```python
from build123d import *

# Parameters (mm, degrees)
F0_R     = 10.16
F1_DEPTH = 15.7734
F2_DEPTH = 40.2336
F3_R     = 3.302


with BuildPart() as f1:
    # F0 (on Top) → F1 (new body)
    with BuildSketch(Plane.XY):
        with BuildLine():
            ThreePointArc((5.403247, 28.0595), (22.033252, 18.195231), (28.575, 0))
            ThreePointArc((28.575, 0), (22.033252, -18.195231), (5.403247, -28.0595))
            Line((5.403247, -28.0595), (53.975, -18.706333))
            ThreePointArc((53.975, -18.706333), (69.422835, 0), (53.975, 18.706333))
            Line((53.975, 18.706333), (5.403247, 28.0595))
        make_face()
        with Locations((53.975, 0)):
            Circle(F0_R, mode=Mode.SUBTRACT)
    extrude(amount=F1_DEPTH)

    # F0 (on Top) → F2 (join)
    with BuildSketch(Plane.XY):
        with BuildLine():
            ThreePointArc((5.403247, -28.0595), (22.033252, -18.195231), (28.575, 0))
            ThreePointArc((28.575, 0), (22.033252, 18.195231), (5.403247, 28.0595))
            ThreePointArc((5.403247, 28.0595), (-28.575, 0), (5.403247, -28.0595))
        make_face()
        with BuildLine():
            ThreePointArc((13.447765, -4.826), (-14.2875, 0), (13.447765, 4.826))
            Line((13.447765, 4.826), (18.5293, 4.826))
            Line((18.5293, 4.826), (18.5293, 0))
            Line((18.5293, 0), (18.5293, -4.826))
            Line((18.5293, -4.826), (13.447765, -4.826))
        make_face(mode=Mode.SUBTRACT)
    extrude(amount=F2_DEPTH)

    # F3
    f3_edges = [f1.edges().sort_by_distance(p)[0] for p in [
        (-5.403247, 28.0595, 40.2336),
    ]]
    fillet(f3_edges, radius=F3_R)


solid = f1.part
```
Source: CAD feature listing. Evaluate the final solid. Frame: model axes, mm. A direction names the side the tool comes from. Give positions to 0.01 mm unless a question says otherwise; leave off trailing zeros. Order: outer loops, then holes, each group sorted by start corner. A loop starts at its lowest first (then second) coordinate and runs counter-clockwise, first axis right, second up.
(1) Pull-direction query (Y, two-part tool) for faces 1 (the face through (16, 4.826, 20)), 2 (the face through (20, 0, 0)), 3 (the face through (69.42, -0.37, 7.78)), 4 (the face through (29.35, -23.45, 7.78)); classes: +Y half, -Y half, draft (parallel to the pull), parting line (faces both ways), or undercut.
(2) Material intervals for line 1 along X through (y, z) = (-0.5, 10.5); line 2 along Y through (x, z) = (0, 18) (1 decimal); line 3 along Z through (x, y) = (35, -4), sorted ascending.
(3) Contact query for flat-ended pins moving along their axis: P1, Ø1.5, axis at x = 16, z = 19.5, coming from the +Y side; P2, Ø5, axis at y = -12.5, z = 6, coming from the +X side; P3, Ø5, axis at y = -18, z = 15.5, coming from the +X side. Output: stop coordinate, or through.
(4) Access query for faces 5 (the face through (30.029, 23.317, 7.776)), 6 (the face through (16, -4.826, 20)). Directions: +Z, -Z, +X, -X, +Y, -Y. A direction counts if a zero-diameter tool reaches every point of the face in a straight line with its end or side. Return the directions, or none.
(5) Section query D-D (x = 37). Return the cut outline in (y, z), plus the area to 3 significant figures.
(6) Section query A-A (z = 6.5). State how many separate pieces and enclosed holes the cut face has, plus the area to 3 significant figures.
Outcome:
1. face 1: undercut
1. face 2: draft
1. face 3: parting line
1. face 4: -Y half
2. line 1: x = -28.57 to -14.28, 18.53 to 43.83, 64.12 to 69.42
2. line 2: y = -28.6 to -14.3, 14.3 to 28.6
2. line 3: z = 0 to 15.77
3. P1: stops at y = 24.17
3. P2: stops at x = 66.59
3. P3: stops at x = 61.45
4. face 5: +Z, -Z, +X, +Y
4. face 6: +Z, -Z
5. outline: (-21.98, 0) - (21.98, 0) - (21.98, 15.77) - (-21.98, 15.77) - close
5. area: 693 mm2
6. separate pieces: 1
6. enclosed holes: 2
6. area: 3,290 mm2
